```python
from build123d import *

# Parameters (mm, degrees)
SKETCH_1_W          = 15
SKETCH_1_H          = 15
SKETCH_1_R          = 2
EXTRUDE_1_DEPTH     = 15
SKETCH_2_R          = 2
CUT_EXTRUDE_1_DEPTH = 15
SKETCH_3_R          = 2
CUT_EXTRUDE_2_DEPTH = 15


with BuildPart() as part:
    # 草图1 → 凸台-拉伸1 (new body)
    with BuildSketch(Plane(origin=(0, 0, 0), x_dir=(1, 0, 0), z_dir=(0, 1, 0))):
        Rectangle(SKETCH_1_W, SKETCH_1_H)
        with Locations(Location((0, 0, 0), (0, 0, 270))):
            Circle(SKETCH_1_R, mode=Mode.SUBTRACT)
    extrude(amount=EXTRUDE_1_DEPTH)

    # 草图2 → 切除-拉伸1 (cut)
    with BuildSketch(Plane.XY.offset(7.5)):
        with Locations((0, 7.5)):
            Circle(SKETCH_2_R)
    extrude(amount=-CUT_EXTRUDE_1_DEPTH, mode=Mode.SUBTRACT)

    # 草图3 → 切除-拉伸2 (cut)
    with BuildSketch(Plane.ZY.offset(7.5)):
        with Locations((0, 7.5)):
            Circle(SKETCH_3_R)
    extrude(amount=-CUT_EXTRUDE_2_DEPTH, mode=Mode.SUBTRACT)


solid = part.part
```
Check sheet for the modelled part. Datum: model origin and axes. Units: mm. Give positions to 0.01 mm unless a question says otherwise; leave off trailing zeros. Write each loop counter-clockwise with the first axis right and the second up, starting at its lowest first coordinate (ties: lowest second). Pieces come first, ordered by that corner, then holes. Notation, with made-up numbers: (54, 2) - (104, 2) arc R33 ccw to (104, 35) - close; hole circle Ø3 at (30, 49). An arc over 180 degrees is marked (long way). Answer as a JSON object with one key per item and string values. Group by question number.
1) Sectioned sample at C-C (z = -5.25). Record the cut outline in (x, y).
2) Sectioned sample at D-D (x = 5.75). Record the cut outline in (y, z).
3) Sectioned sample at A-A (y = 7.5). Record the cut outline in (x, z).
4) Depth check by flat-ended pin: P1, Ø2, axis at x = 1, z = 3.5, coming from the -Y side. Enter the tip coordinate at first touch or a pass-through.
5) Sectioned sample at B-B (x = 0). Record the cut outline in (y, z), then the cut area to 3 significant figures.
6) Release check for a two-part mould opening along X. For faces 1 (the face through (1.352, 11.915, -1.474)), 2 (the face through (-2, 0, -2)), 3 (the face through (-1.998, 7.588, 4.5)), 4 (the face through (-7.5, 9, 2)) record: pulls with the +X half, pulls with the -X half, needs draft (parallel to the pull), parting line crosses it, or undercut.
7) Thickness scan on probe 1 along Y at (x, z) = (-3.5, 0); probe 2 along Z at (x, y) = (0, 13). Record the ranges inside material, lowest first. Write a range as from..to.
Geometry results:
{
 "1": {"outline": "(-7.5, 0) - (7.5, 0) - (7.5, 15) - (-7.5, 15) - close; hole circle Ø4 at (0, 7.5)"},
 "2": {"outline": "(0, -7.5) - (15, -7.5) - (15, 7.5) - (0, 7.5) - close; hole circle Ø4 at (7.5, 0)"},
 "3": {"outline": "(-7.5, -7.5) - (-2, -7.5) - (-2, -2) - (-7.5, -2) - close; (-7.5, 2) - (-2, 2) - (-2, 7.5) - (-7.5, 7.5) - close; (2, -7.5) - (7.5, -7.5) - (7.5, -2) - (2, -2) - close; (2, 2) - (7.5, 2) - (7.5, 7.5) - (2, 7.5) - close"},
 "4": {"P1": "stops at y = 0"},
 "5": {"outline": "(0, -7.5) - (5.5, -7.5) - (5.5, -2) - (0, -2) - close; (0, 2) - (5.5, 2) - (5.5, 7.5) - (0, 7.5) - close; (9.5, -7.5) - (15, -7.5) - (15, -2) - (9.5, -2) - close; (9.5, 2) - (15, 2) - (15, 7.5) - (9.5, 7.5) - close", "area": "121 mm^2"},
 "6": {"face 1": "undercut", "face 2": "needs draft", "face 3": "undercut", "face 4": "pulls with the -X half"},
 "7": {"probe 1": "y = 0..5.5, 9.5..15", "probe 2": "z = -7.5..-2, 2..7.5"}
}
